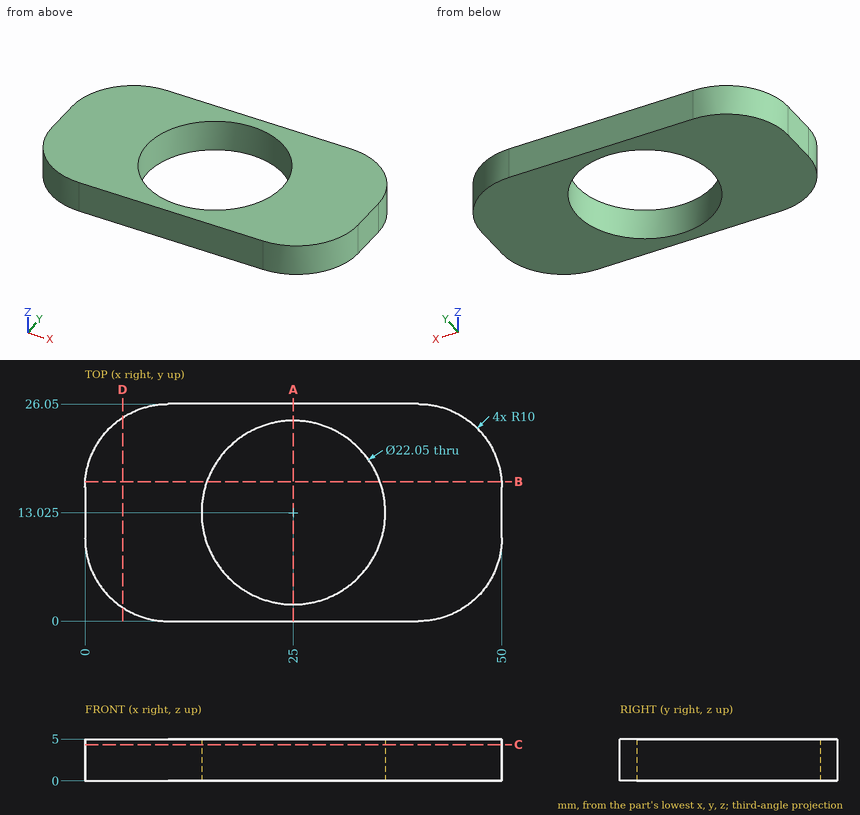
Input: dimensioned drawing with shaded views. Units: mm. Origin: part minimum x, y, z. Give positions to 0.01 mm unless a question says otherwise; leave off trailing zeros. Loops run counter-clockwise (first coordinate to the right, second up) from the corner with the lowest first, then second, coordinate; pieces in that order, holes last. Notation, with made-up numbers: M 60,32 L 99,32 A23 cw 99,59 Z; hole C 33.5,-2.5 d3. An arc over 180 degrees is marked long. Put each result on its own line as item: value.
1) Material intervals for L1, parallel to Y at x = 25, z = 3.3; L2, parallel to X at y = 13.25, z = 3.5; L3, parallel to X at y = 17.5, z = 0.9, sorted ascending. Write a range as from..to.
Computed values:
L1: y = 0..2, 24.05..26.05
L2: x = 0..13.98, 36.02..50
L3: x = 0.11..14.92, 35.08..49.89
2) Cut plane D-D, the plane x = 4.5. Return the cut outline in (y, z), plus the area to 3 significant figures.
Computed values:
outline: M 1.65,0 L 24.4,0 L 24.4,5 L 1.65,5 Z
area: 114 mm^2
3) First-contact query: P1, Ø2, axis at y = 5, z = 1.5, coming from the +X side; P2, Ø3, axis at y = 8, z = 1, coming from the -X side. Flat tips, straight axial feed; report the tip coordinate or a pass-through.
Computed values:
P1: stops at x = 49.17
P2: stops at x = 0.01
4) Cut plane B-B, the plane y = 16.75. Return the cut outline in (x, z), plus the area to 3 significant figures.
Computed values:
outline: M 0.02,0 L 14.62,0 L 14.62,5 L 0.02,5 Z; M 35.38,0 L 49.98,0 L 49.98,5 L 35.38,5 Z
area: 146 mm^2
5) Cut plane C-C, the plane z = 4.35. Return the cut outline in (x, y) (3 decimals).
Computed values:
outline: M 0,10 A10 ccw 10,0 L 40,0 A10 ccw 50,10 L 50,16.05 A10 ccw 40,26.05 L 10,26.05 A10 ccw 0,16.05 Z; hole C 25,13.025 d22.05
6) Cut plane A-A, the plane x = 25. Return the cut outline in (y, z).
Computed values:
outline: M 0,0 L 2,0 L 2,5 L 0,5 Z; M 24.05,0 L 26.05,0 L 26.05,5 L 24.05,5 Z
